Work out the finished part from the listing and answer in its coordinate system (mm). Face numbers are marked on the shaded views. Round coordinates to 2 decimals unless told otherwise and drop trailing zeros. Loops run counter-clockwise (first coordinate to the right, second up) from the corner with the lowest first, then second, coordinate; pieces in that order, holes last. Notation, with made-up numbers: M 3.25,76.25 L 60.25,76.25 A11 cw 60.25,87.25 Z; hole C 31.25,86 d8. An arc over 180 degrees is marked long. One line per item, written item: value.
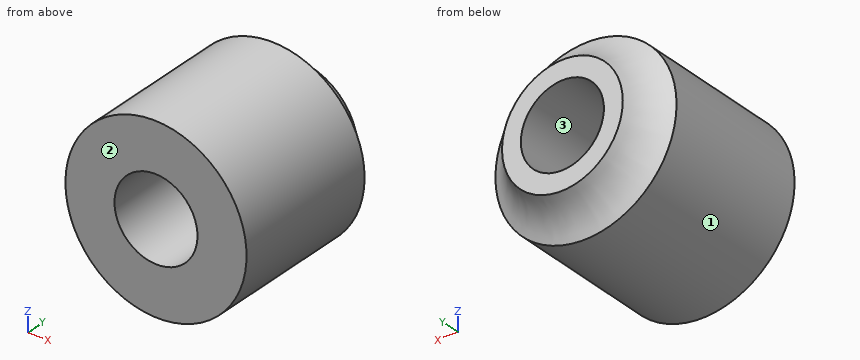
Autodesk Inventor part; units mm, degrees
ref_plane "YZ Plane" through (0, 0, 0) normal (1, 0, 0) x (0, 1, 0)
ref_plane "XZ Plane" through (0, 0, 0) normal (0, 1, 0) x (-1, 0, 0)
ref_plane "XY Plane" through (0, 0, 0) normal (0, 0, 1) x (1, 0, 0)
sketch "Sketch1" plane through (0, 0, 0) normal (0, 1, 0) x (-1, 0, 0)
  circle A0 centre (0, 0) radius 6
  circle A1 centre (0, 0) radius 2.75
  dimension "d0" = 12
  dimension "d1" = 5.5
extrude "Extrusion1" add sketch "Sketch1" along normal blind 10
sketch "Sketch2" plane through (0, 10, 0) normal (0, 1, 0) x (1, 0, 0)
  circle A0 centre (0, 0) radius 2.75
  circle A1 centre (0, 0) radius 4
  dimension "d4" = 5.5
  dimension "d5" = 8
extrude "Extrusion2" add sketch "Sketch2" along normal blind 2
fillet "Fillet1" radius 4 1 edges at (-4, 10, 0)
properties part number "Idler_Spacer"
1) Find the intervals of material crossed by probe 1 along X at (y, z) = (2.5, 0); probe 2 along X at (y, z) = (7.5, -2.25), in increasing order. Write a range as from..to.
Check values:
probe 1: -6..-2.75, 2.75..6
probe 2: -5.56..-1.58, 1.58..5.56
2) The mould has two halves that part along X. Classify the marked faces 1, 2 and 3: +X half, -X half, draft (parallel to the pull), parting line (faces both ways), or undercut.
Check values:
face 1: parting line
face 2: draft
face 3: undercut
3) Find section A-A (y = 2.75). Give the vertices of the cut face in (x, z).
Check values:
outline: C 0,0 d12; hole C 0,0 d5.5
4) This flat-tipped pin is pushed along its axis until it touches: pin 1 (1 mm diameter, centred on x = -2.5, y = 10, fed in from -Z). Where does it stop, or does it pass through?
Check values:
pin 1: z = -5.66
